from build123d import *

# Parameters (mm, degrees)
SKETCH_1_W          = 111
SKETCH_1_H          = 124
SKETCH_1_R          = 2.6
SKETCH_1_R_2        = 1.6
EXTRUDE_1_DEPTH     = 3
SKETCH_2_R          = 1.6
CUT_EXTRUDE_1_DEPTH = 84.266139577
CUT_EXTRUDE_3_DEPTH = 84.266139577
CUT_EXTRUDE_4_DEPTH = 84.266139577
FILLET_1_R          = 8
FILLET_2_R          = 3
FILLET_3_R          = 5


with BuildPart() as part:
    # 草图1 → 凸台-拉伸1 (new body)
    with BuildSketch(Plane.XY):
        Rectangle(SKETCH_1_W, SKETCH_1_H)
        with Locations((-30, -57)):
            Circle(SKETCH_1_R, mode=Mode.SUBTRACT)
        with Locations((-50.5, -57)):
            Circle(SKETCH_1_R_2, mode=Mode.SUBTRACT)
        with Locations(Location((30, -57, 0), (0, 0, 180))):
            Circle(SKETCH_1_R, mode=Mode.SUBTRACT)
        with Locations(Location((50.5, -57, 0), (0, 0, 180))):
            Circle(SKETCH_1_R_2, mode=Mode.SUBTRACT)
    extrude(amount=EXTRUDE_1_DEPTH)

    # 草图2 → 切除-拉伸1 (cut, through all)
    with BuildSketch(Plane.XY.offset(3)):
        with Locations((-52.5, 22)):
            Circle(SKETCH_2_R)
        with Locations((-52.5, 42)):
            Circle(SKETCH_2_R)
        with Locations((-52.5, 32)):
            Circle(SKETCH_2_R)
        with Locations((-52.5, 52)):
            Circle(SKETCH_2_R)
        with Locations((-52.5, 12)):
            Circle(SKETCH_2_R)
        with Locations(Location((52.5, 12, 0), (0, 0, 180))):
            Circle(SKETCH_2_R)
        with Locations(Location((52.5, 52, 0), (0, 0, 180))):
            Circle(SKETCH_2_R)
        with Locations(Location((52.5, 32, 0), (0, 0, 180))):
            Circle(SKETCH_2_R)
        with Locations(Location((52.5, 42, 0), (0, 0, 180))):
            Circle(SKETCH_2_R)
        with Locations(Location((52.5, 22, 0), (0, 0, 180))):
            Circle(SKETCH_2_R)
    extrude(amount=-CUT_EXTRUDE_1_DEPTH, mode=Mode.SUBTRACT)

    # 草图5 → 切除-拉伸3 (cut, through all)
    with BuildSketch(Plane(origin=(0, 0, 0), x_dir=(-1, 0, 0), z_dir=(0, 0, -1))):
        Polygon((-32, 62), (-18, 10), (18, 10), (32, 62), align=None)
    extrude(amount=-CUT_EXTRUDE_3_DEPTH, mode=Mode.SUBTRACT)

    # 草图6 → 切除-拉伸4 (cut, through all)
    with BuildSketch(Plane(origin=(0, 0, 0), x_dir=(-1, 0, 0), z_dir=(0, 0, -1))):
        Polygon((-45.5, 52), (-45.5, 32), (-30.136728624, 32), (-35.521344008, 52), align=None)
        Polygon((-45.5, 1.976583298), (-23.638160979, 7.862463034), (-28.790574777, 27), (-45.5, 27), align=None)
        Polygon((-0.923076923, 4), (-22.598267085, 4), (-45.5, -2.165851169), (-45.5, -13), (-5.5, -13), align=None)
        Polygon((45.5, -2.165851169), (22.598267085, 4), (0.923076923, 4), (5.5, -13), (45.5, -13), align=None)
        Polygon((28.790574777, 27), (23.638160979, 7.862463034), (45.5, 1.976583298), (45.5, 27), align=None)
        Polygon((35.521344008, 52), (45.5, 52), (45.5, 32), (30.136728624, 32), align=None)
        Polygon((45.5, -46), (45.5, -18), (6.846153846, -18), (14.384615385, -46), align=None)
        Polygon((-45.5, -18), (-6.846153846, -18), (-14.384615385, -46), (-45.5, -46), align=None)
        Polygon((10.552726147, -51), (0, -11.804160025), (0, -51), align=None)
        Polygon((0, -51), (0, -11.804160025), (-10.552726147, -51), align=None)
    extrude(amount=-CUT_EXTRUDE_4_DEPTH, mode=Mode.SUBTRACT)

    # 圆角1
    fillet_1_edges = [part.edges().sort_by_distance(p)[0] for p in [
        (0.923076923, 4, 1.5),
        (-0.923076923, 4, 1.5),
    ]]
    fillet(fillet_1_edges, radius=FILLET_1_R)

    # 圆角2
    fillet_2_edges = [part.edges().sort_by_distance(p)[0] for p in [
        (45.5, -2.165851169, 1.5),
        (22.598267085, 4, 1.5),
        (5.5, -13, 1.5),
        (45.5, -13, 1.5),
        (45.5, 1.976583298, 1.5),
        (45.5, 27, 1.5),
        (28.790574777, 27, 1.5),
        (23.638160979, 7.862463034, 1.5),
        (-45.5, 1.976583298, 1.5),
        (-23.638160979, 7.862463034, 1.5),
        (-28.790574777, 27, 1.5),
        (-45.5, 27, 1.5),
        (-45.5, -2.165851169, 1.5),
        (-45.5, -13, 1.5),
        (-5.5, -13, 1.5),
        (-22.598267085, 4, 1.5),
        (45.5, -18, 1.5),
        (6.846153846, -18, 1.5),
        (14.384615385, -46, 1.5),
        (45.5, -46, 1.5),
        (0, -11.804160025, 1.5),
        (-10.552726147, -51, 1.5),
        (10.552726147, -51, 1.5),
        (-45.5, -18, 1.5),
        (-45.5, -46, 1.5),
        (-14.384615385, -46, 1.5),
        (-6.846153846, -18, 1.5),
        (-35.521344008, 52, 1.5),
        (-45.5, 52, 1.5),
        (-45.5, 32, 1.5),
        (-30.136728624, 32, 1.5),
        (45.5, 32, 1.5),
        (45.5, 52, 1.5),
        (35.521344008, 52, 1.5),
        (30.136728624, 32, 1.5),
    ]]
    fillet(fillet_2_edges, radius=FILLET_2_R)

    # 圆角3
    fillet_3_edges = [part.edges().sort_by_distance(p)[0] for p in [
        (-18, 10, 1.5),
        (18, 10, 1.5),
    ]]
    fillet(fillet_3_edges, radius=FILLET_3_R)


solid = part.part
The listing builds one solid part. Answer for the finished solid, in the listing's coordinates (mm). Give positions to 0.01 mm unless a question says otherwise; leave off trailing zeros. Write each loop counter-clockwise with the first axis right and the second up, starting at its lowest first coordinate (ties: lowest second). Pieces come first, ordered by that corner, then holes.
1) Section C-C (y = 8.5) is taken. Write down the section's boundary in (x, z).
2) Given P1, Ø1.5, axis at x = -6.5, z = 1.5, coming from the +Y side; P2, Ø7, axis at x = 30, y = -57, coming from the +Z side, each flat-ended and moving along its own axis, determine where each tip first touches the part or whether it passes through.
3) Section A-A (y = -34) is taken. Write down the section's boundary in (x, z).
4) Section D-D (y = 22) is taken. Write down the section's boundary in (x, z), and give its area (3 significant figures).
5) Find the intervals of material crossed by L1, parallel to Y at x = -52.5, z = 0.7; L2, parallel to X at y = -8.5, z = 1.35; L3, parallel to X at y = -41, z = 1.65, in increasing order.
6) Section B-B (z = 0.95) is taken. Count the separate pieces of the cut face and the enclosed holes in it, and give its area (3 significant figures).
Response:
1. outline: (-55.5, 0) - (-45.5, 0) - (-45.5, 3) - (-55.5, 3) - close; (-24.71, 0) - (24.71, 0) - (24.71, 3) - (-24.71, 3) - close; (45.5, 0) - (55.5, 0) - (55.5, 3) - (45.5, 3) - close
2. P1: stops at y = 10
2. P2: stops at z = 3
3. outline: (-55.5, 0) - (-45.5, 0) - (-45.5, 3) - (-55.5, 3) - close; (-11.15, 0) - (-5.98, 0) - (-5.98, 3) - (-11.15, 3) - close; (5.98, 0) - (11.15, 0) - (11.15, 3) - (5.98, 3) - close; (45.5, 0) - (55.5, 0) - (55.5, 3) - (45.5, 3) - close
4. outline: (-55.5, 0) - (-54.1, 0) - (-54.1, 3) - (-55.5, 3) - close; (-50.9, 0) - (-45.5, 0) - (-45.5, 3) - (-50.9, 3) - close; (-27.44, 0) - (-21.23, 0) - (-21.23, 3) - (-27.44, 3) - close; (21.23, 0) - (27.44, 0) - (27.44, 3) - (21.23, 3) - close; (45.5, 0) - (50.9, 0) - (50.9, 3) - (45.5, 3) - close; (54.1, 0) - (55.5, 0) - (55.5, 3) - (54.1, 3) - close
4. area: 78.1 mm2
5. L1: y = -62 to 10.4, 13.6 to 20.4, 23.6 to 30.4, 33.6 to 40.4, 43.6 to 50.4, 53.6 to 62
5. L2: x = -55.5 to -45.5, -4.29 to 4.29, 45.5 to 55.5
5. L3: x = -55.5 to -45.5, -13.04 to -7.86, 7.86 to 13.04, 45.5 to 55.5
6. separate pieces: 1
6. enclosed holes: 23
6. area: 6,130 mm2
